Work out the finished part from the listing and answer in its coordinate system (mm). Face numbers are marked on the shaded views. A direction names the side the tool comes from. Coordinates: 2 decimals unless noted, no trailing zeros. Write each loop counter-clockwise with the first axis right and the second up, starting at its lowest first coordinate (ties: lowest second). Pieces come first, ordered by that corner, then holes. Notation, with made-up numbers: M 59,23.25 L 96,23.25 A18 ccw 96,48.25 Z; hole C -28.75,24.5 d7. An arc over 180 degrees is marked long. Answer as CSV lines item,"result". Start each with the question number.
(1) Flat-ended cylindrical pins translate along their axes: P1, Ø2, axis at y = 12.5, z = 1, coming from the -X side; P2, Ø4, axis at x = -6, z = 1.5, coming from the +Y side; P3, Ø3, axis at y = 20, z = 0, coming from the -X side. Find the tip coordinate at first contact, or state that the pin passes through.
(2) For the marked faces 1 and 2, determine the directions among +Z, -Z, +X, -X, +Y, -Y from which every point of the face is accessible in a straight line to the end or side of a thin tool.
(3) A cutting plane is placed at C-C on x = -10. Give the vertices of the cut face in (y, z).
(4) A cutting plane is placed at A-A on y = 10. Give the vertices of the cut face in (x, z).
(5) A cutting plane is placed at D-D on y = 3.5. Give the vertices of the cut face in (x, z), then the cut area to 3 significant figures.
(6) Find the intervals of material crossed by L1, parallel to Y at x = 6.75, z = 0; L2, parallel to Y at x = 1.25, z = 2; L3, parallel to X at y = 17, z = -2, in increasing order. Write a range as [from, to].
(7) A cutting plane is placed at B-B on z = 0. Give the vertices of the cut face in (x, y).
(8) The mould has two halves that part along Z. Classify the marked faces 3, 4, 5 and 6: released by +Z, released by -Z, zero draft, split by the parting line, or undercut.
from build123d import *

# Parameters (mm, degrees)
SKETCH1_W           = 20
SKETCH1_H           = 7.5
SKETCH1_R           = 2
BOSS_EXTRUDE1_DEPTH = 4
SKETCH2_W           = 7.5
SKETCH2_H           = 25
SKETCH2_R           = 2
BOSS_EXTRUDE2_DEPTH = 5


with BuildPart() as part:
    # Sketch1 → Boss-Extrude1 (new body)
    with BuildSketch(Plane(origin=(0, 0, 0), x_dir=(1, 0, 0), z_dir=(0, 1, 0))):
        with Locations((-5, 0)):
            Rectangle(SKETCH1_W, SKETCH1_H)
        with Locations(Location((0, 0, 0), (0, 0, 270))):
            Circle(SKETCH1_R, mode=Mode.SUBTRACT)
        with Locations(Location((-10, 0, 0), (0, 0, 270))):
            Circle(SKETCH1_R, mode=Mode.SUBTRACT)
    extrude(amount=BOSS_EXTRUDE1_DEPTH)

    # Sketch2 → Boss-Extrude2 (add)
    with BuildSketch(Plane(origin=(5, 0, 0), x_dir=(0, 0, -1), z_dir=(1, 0, 0))):
        with Locations((0, 12.5)):
            Rectangle(SKETCH2_W, SKETCH2_H)
        with Locations((0, 20)):
            Circle(SKETCH2_R, mode=Mode.SUBTRACT)
        with Locations((0, 10)):
            Circle(SKETCH2_R, mode=Mode.SUBTRACT)
    extrude(amount=BOSS_EXTRUDE2_DEPTH)


solid = part.part
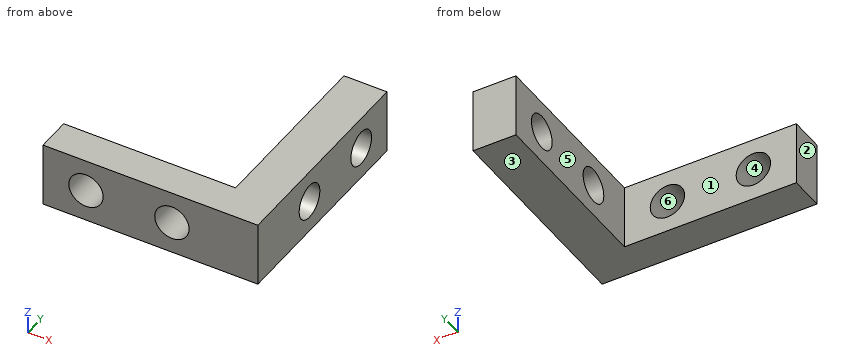
Here are the results:
1,P1,"stops at x = 5"
1,P2,"stops at y = 4"
1,P3,"passes through"
2,face 1,"+Z, -Z, -X, +Y"
2,face 2,"+Z, -Z, -X, +Y, -Y"
3,outline,"M 0,-3.75 L 4,-3.75 L 4,-2 L 0,-2 Z; M 0,2 L 4,2 L 4,3.75 L 0,3.75 Z"
4,outline,"M 5,-3.75 L 10,-3.75 L 10,-2 L 5,-2 Z; M 5,2 L 10,2 L 10,3.75 L 5,3.75 Z"
5,outline,"M -15,-3.75 L 10,-3.75 L 10,3.75 L -15,3.75 Z; hole C -10,0 d4; hole C 0,0 d4"
5,area,"162 mm^2"
6,L1,"y = [0, 8], [12, 18], [22, 25]"
6,L2,"y = [0, 4]"
6,L3,"x = [5, 10]"
7,outline,"M -15,0 L -12,0 L -12,4 L -15,4 Z; M -8,0 L -2,0 L -2,4 L -8,4 Z; M 2,0 L 10,0 L 10,8 L 5,8 L 5,4 L 2,4 Z; M 5,12 L 10,12 L 10,18 L 5,18 Z; M 5,22 L 10,22 L 10,25 L 5,25 Z"
8,face 3,"released by -Z"
8,face 4,"undercut"
8,face 5,"zero draft"
8,face 6,"undercut"
